Input: part model. Units: mm. Frame: model coordinates. Face numbers are marked on the shaded views. A direction names the side the tool comes from. Coordinates: 2 decimals unless noted, no trailing zeros. Write each loop counter-clockwise with the first axis right and the second up, starting at its lowest first coordinate (ties: lowest second). Pieces come first, ordered by that corner, then holes. Notation, with made-up numbers: M 49.25,65 L 57.25,65 A19 ccw 57.25,84 Z; hole C 24,47 d11. An arc over 180 degrees is marked long. Use CSV: the item, a comma, the result in double quotes.
Autodesk Inventor part; units mm, degrees
ref_plane "YZ Plane" through (0, 0, 0) normal (1, 0, 0) x (0, 1, 0)
ref_plane "XZ Plane" through (0, 0, 0) normal (0, 1, 0) x (-1, 0, 0)
ref_plane "XY Plane" through (0, 0, 0) normal (0, 0, 1) x (1, 0, 0)
sketch "スケッチ1" plane through (0, 0, 0) normal (0, 0, 1) x (1, 0, 0)
  line L0 (0, 0) -> (10, 0)
  line L1 (10, 0) -> (10, 130)
  line L2 (10, 130) -> (0, 130)
  line L3 (0, 130) -> (0, 0)
  dimension "d0" = 10
  dimension "d1" = 130
extrude "押し出し1" add sketch "スケッチ1" along normal blind 20
sketch "スケッチ2" plane through (0, 0, 20) normal (0, 0, 1) x (1, 0, 0)
  line L0 (10, 130) -> (0, 130)
  line L1 (5, 130) -> (5, 0) construction
  line L2 (0, 0) -> (10, 0)
  point P0 (5, 5)
  point P1 (5, 32)
  dimension "d4" = 27
  dimension "d5" = 5
hole "穴1" at (5, 5, 20) at (5, 32, 20) direction (0, 0, -1) diameter 4.2 depth 20
sketch "スケッチ3" plane through (10, 0, 0) normal (1, 0, 0) x (0, 0, -1)
  line L0 (-20, 0) -> (-20, 130)
  line L1 (0, 0) -> (0, 130)
  line L2 (-20, 120) -> (0, 120)
  line L3 (0, 120) -> (0, 40)
  line L4 (0, 40) -> (-20, 40)
  line L5 (-20, 40) -> (-20, 120)
  line L6 (0, 130) -> (-20, 130)
  point P0 (-10, 120)
  point P1 (-20, 40)
  point P2 (0, 120)
  dimension "d13" = 10
  dimension "d14" = 80
extrude "押し出し2" cut sketch "スケッチ3" against normal blind 5 contours L0 L2 L1 L4
fillet "フィレット1" radius 4 4 edges at (10, 0, 10) (0, 0, 10) (10, 130, 10) (0, 130, 10)
properties part number "finger1" material "アセタール樹脂、白"
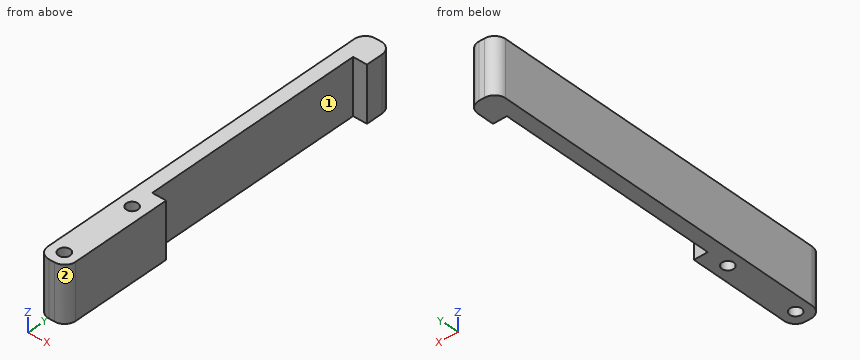
1. Section A-A (y = 32). Return loops of the section in (x, z).
Resolved:
outline,"M 0,0 L 2.9,0 L 2.9,20 L 0,20 Z; M 7.1,0 L 10,0 L 10,20 L 7.1,20 Z"
2. Access query for the marked faces 1 and 2. Directions: +Z, -Z, +X, -X, +Y, -Y. A direction counts if a zero-diameter tool reaches every point of the face in a straight line with its end or side. Return the directions, or none.
Resolved:
face 1,"+Z, -Z, +X"
face 2,"+Z, -Z, +X, -Y"
3. Section B-B (z = 7.5). Return loops of the section in (x, y), then the cut area to 3 significant figures.
Resolved:
outline,"M 0,4 A4 ccw 4,0 L 6,0 A4 ccw 10,4 L 10,40 L 5,40 L 5,120 L 10,120 L 10,126 A4 ccw 6,130 L 4,130 A4 ccw 0,126 Z; hole C 5,5 d4.2; hole C 5,32 d4.2"
area,"859 mm^2"
4. Contact query for flat-ended pins moving along their axis: pin 1 Ø2 at (x, z) = (1.5, 9.5) entering from +Y; pin 2 Ø1.5 at (x, z) = (3, 10) entering from +Y; pin 3 Ø4 at (y, z) = (93.5, 4) entering from +X; pin 4 Ø4 at (x, y) = (5, 5) entering from +Z. Output: stop coordinate, or through.
Resolved:
pin 1,"stops at y = 129.71"
pin 2,"stops at y = 129.99"
pin 3,"stops at x = 5"
pin 4,"passes through"
5. Material intervals for line 1 (Y direction, x = 6.5, z = 15); line 2 (Y direction, x = 4, z = 2); line 3 (X direction, y = 32, z = 6.5), sorted ascending. Write a range as [from, to].
Resolved:
line 1,"y = [0.03, 3.53], [6.47, 30.53], [33.47, 40], [120, 129.97]"
line 2,"y = [0, 3.15], [6.85, 30.15], [33.85, 130]"
line 3,"x = [0, 2.9], [7.1, 10]"
6. Section C-C (x = 1.25). Return loops of the section in (y, z), then the cut area to 3 significant figures.
Resolved:
outline,"M 1.1,0 L 128.9,0 L 128.9,20 L 1.1,20 Z"
area,"2,560 mm^2"
